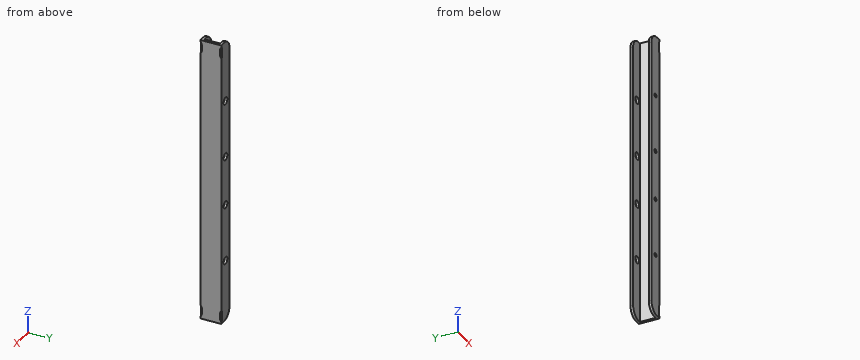
```python
from build123d import *

# Parameters (mm, degrees)
BOSS_EXTRUDE1_DEPTH = 174.625
CUT_EXTRUDE1_REACH  = 179.488
SKETCH3_R           = 2.3495
CUT_EXTRUDE2_REACH  = 179.488
SKETCH4_R           = 4.3688
FILLET1_R           = 12.7


with BuildPart() as part:
    # Sketch1 → Boss-Extrude1 (new, symmetric)
    with BuildSketch(Plane.XY):
        Polygon((-19.05, 0), (0, 0), (0, 25.4), (-19.05, 25.4), (-19.05, 22.225), (-3.175, 22.225), (-3.175, 3.175), (-19.05, 3.175), align=None)
    extrude(amount=BOSS_EXTRUDE1_DEPTH, both=True)

    # Sketch3 → Cut-Extrude1 (cut, up to next)
    with BuildSketch(Plane.XZ, mode=Mode.PRIVATE) as cut_extrude1_sk1:
        with Locations(Location((-9.525, -30.1752, 0), (0, 0, 270))):
            Circle(SKETCH3_R)
    cut_extrude1_tool1 = extrude(cut_extrude1_sk1.sketch, amount=-CUT_EXTRUDE1_REACH, mode=Mode.PRIVATE) & part.part
    # Sketch3 → Cut-Extrude1 (cut, up to next)
    with BuildSketch(Plane.XZ, mode=Mode.PRIVATE) as cut_extrude1_sk2:
        with Locations(Location((-9.525, -100.0252, 0), (0, 0, 270))):
            Circle(SKETCH3_R)
    cut_extrude1_tool2 = extrude(cut_extrude1_sk2.sketch, amount=-CUT_EXTRUDE1_REACH, mode=Mode.PRIVATE) & part.part
    # Sketch3 → Cut-Extrude1 (cut, up to next)
    with BuildSketch(Plane.XZ, mode=Mode.PRIVATE) as cut_extrude1_sk3:
        with Locations(Location((-9.525, 30.1752, 0), (0, 0, 270))):
            Circle(SKETCH3_R)
    cut_extrude1_tool3 = extrude(cut_extrude1_sk3.sketch, amount=-CUT_EXTRUDE1_REACH, mode=Mode.PRIVATE) & part.part
    # Sketch3 → Cut-Extrude1 (cut, up to next)
    with BuildSketch(Plane.XZ, mode=Mode.PRIVATE) as cut_extrude1_sk4:
        with Locations(Location((-9.525, 100.0252, 0), (0, 0, 270))):
            Circle(SKETCH3_R)
    cut_extrude1_tool4 = extrude(cut_extrude1_sk4.sketch, amount=-CUT_EXTRUDE1_REACH, mode=Mode.PRIVATE) & part.part
    add(cut_extrude1_tool1.solids().sort_by_distance((-9.525, 0, -30.1752))[0], mode=Mode.SUBTRACT)
    add(cut_extrude1_tool2.solids().sort_by_distance((-9.525, 0, -100.0252))[0], mode=Mode.SUBTRACT)
    add(cut_extrude1_tool3.solids().sort_by_distance((-9.525, 0, 30.1752))[0], mode=Mode.SUBTRACT)
    add(cut_extrude1_tool4.solids().sort_by_distance((-9.525, 0, 100.0252))[0], mode=Mode.SUBTRACT)

    # Sketch4 → Cut-Extrude2 (cut, up to next)
    with BuildSketch(Plane(origin=(0, 25.4, 0), x_dir=(1, 0, 0), z_dir=(0, 1, 0)), mode=Mode.PRIVATE) as cut_extrude2_sk1:
        with Locations(Location((-9.525, -100.0252, 0), (0, 0, 180))):
            Circle(SKETCH4_R)
    cut_extrude2_tool1 = extrude(cut_extrude2_sk1.sketch, amount=-CUT_EXTRUDE2_REACH, mode=Mode.PRIVATE) & part.part
    # Sketch4 → Cut-Extrude2 (cut, up to next)
    with BuildSketch(Plane(origin=(0, 25.4, 0), x_dir=(1, 0, 0), z_dir=(0, 1, 0)), mode=Mode.PRIVATE) as cut_extrude2_sk2:
        with Locations(Location((-9.525, -30.1752, 0), (0, 0, 180))):
            Circle(SKETCH4_R)
    cut_extrude2_tool2 = extrude(cut_extrude2_sk2.sketch, amount=-CUT_EXTRUDE2_REACH, mode=Mode.PRIVATE) & part.part
    # Sketch4 → Cut-Extrude2 (cut, up to next)
    with BuildSketch(Plane(origin=(0, 25.4, 0), x_dir=(1, 0, 0), z_dir=(0, 1, 0)), mode=Mode.PRIVATE) as cut_extrude2_sk3:
        with Locations(Location((-9.525, 30.1752, 0), (0, 0, 180))):
            Circle(SKETCH4_R)
    cut_extrude2_tool3 = extrude(cut_extrude2_sk3.sketch, amount=-CUT_EXTRUDE2_REACH, mode=Mode.PRIVATE) & part.part
    # Sketch4 → Cut-Extrude2 (cut, up to next)
    with BuildSketch(Plane(origin=(0, 25.4, 0), x_dir=(1, 0, 0), z_dir=(0, 1, 0)), mode=Mode.PRIVATE) as cut_extrude2_sk4:
        with Locations(Location((-9.525, 100.0252, 0), (0, 0, 180))):
            Circle(SKETCH4_R)
    cut_extrude2_tool4 = extrude(cut_extrude2_sk4.sketch, amount=-CUT_EXTRUDE2_REACH, mode=Mode.PRIVATE) & part.part
    add(cut_extrude2_tool1.solids().sort_by_distance((-9.525, 25.4, 100.0252))[0], mode=Mode.SUBTRACT)
    add(cut_extrude2_tool2.solids().sort_by_distance((-9.525, 25.4, 30.1752))[0], mode=Mode.SUBTRACT)
    add(cut_extrude2_tool3.solids().sort_by_distance((-9.525, 25.4, -30.1752))[0], mode=Mode.SUBTRACT)
    add(cut_extrude2_tool4.solids().sort_by_distance((-9.525, 25.4, -100.0252))[0], mode=Mode.SUBTRACT)

    # Fillet1
    fillet1_edges = [part.edges().sort_by_distance(p)[0] for p in [
        (-19.05, 1.5875, -174.625),
        (-19.05, 23.8125, 174.625),
        (-19.05, 1.5875, 174.625),
        (-19.05, 23.8125, -174.625),
    ]]
    fillet(fillet1_edges, radius=FILLET1_R)

    # Cut-Sweep1: sweep along a path in Sketch5
    with BuildLine(Plane(origin=(0, 25.4, 0), x_dir=(1, 0, 0), z_dir=(0, 1, 0))) as cut_sweep1_path:
        Line((7.112, -155.829), (4.572, -155.829))
        ThreePointArc((4.572, -155.829), (0.081871939, -157.688871939), (-1.778, -162.179))
        Line((-1.778, -162.179), (-1.778, -168.021))
        ThreePointArc((-1.778, -168.021), (0.081871939, -172.511128061), (4.572, -174.371))
        Line((4.572, -174.371), (7.112, -174.371))
    # Sketch6 → Cut-Sweep1 (sweep, cut)
    with BuildSketch(Plane(origin=(7.112, 25.4, 174.371), x_dir=(0, 0, -1), z_dir=(1, 0, 0))):
        Polygon((-0.508, 0.508), (4.572, -4.572), (4.572, 0.508), align=None)
        Polygon((4.572, -20.828), (4.572, -25.908), (-0.508, -25.908), align=None)
    cut_sweep1 = sweep(path=cut_sweep1_path.line, mode=Mode.SUBTRACT)

    # Mirror1: Cut-Sweep1 across plane
    add(cut_sweep1.mirror(Plane.XY), mode=Mode.SUBTRACT)


solid = part.part
```
Source: CAD feature listing. Evaluate the final solid. Frame: model axes, mm. Coordinates: 2 decimals unless noted, no trailing zeros. Loops run counter-clockwise (first coordinate to the right, second up) from the corner with the lowest first, then second, coordinate; pieces in that order, holes last. Notation, with made-up numbers: (-19, 84) -> (18, 84) arc R8 ccw to (18, 88) -> close; hole circle Ø7 at (55.5, 16). An arc over 180 degrees is marked (long way). One line per item, written item: value. Start each with the question number.
Q1. Contact query for flat-ended pins moving along their axis: P1, Ø8, axis at x = -9.52, z = -30.18, coming from the +Y side (3 decimals); P2, Ø9.5, axis at y = 12.5, z = 70, coming from the -X side (3 decimals); P3, Ø8, axis at x = -12, y = 18.5, coming from the +Z side. Output: stop coordinate, or through.
Q2. Section query B-B, the plane y = 14. Return the cut outline in (x, z) (3 decimals), and give its area (3 significant figures).
Q3. Section query A-A, the plane z = -88.5. Return the cut outline in (x, y) (3 decimals), and give its area (3 significant figures).
Q4. Line query: line 1 along Y through (x, z) = (-10, 36.5) (3 decimals); line 2 along X through (y, z) = (22, -63.5) (3 decimals). Output: solid intervals per line, ascending.
Results:
1. P1: y = 3.175
1. P2: x = -3.175
1. P3: z = 173.91
2. outline: (-3.175, -174.625) -> (0, -174.625) -> (0, 174.625) -> (-3.175, 174.625) -> close
2. area: 1,110 mm^2
3. outline: (-19.05, 0) -> (0, 0) -> (0, 25.4) -> (-19.05, 25.4) -> (-19.05, 22.225) -> (-3.175, 22.225) -> (-3.175, 3.175) -> (-19.05, 3.175) -> close
3. area: 181 mm^2
4. line 1: 0 to 3.175, 22.225 to 25.4
4. line 2: -3.175 to 0
